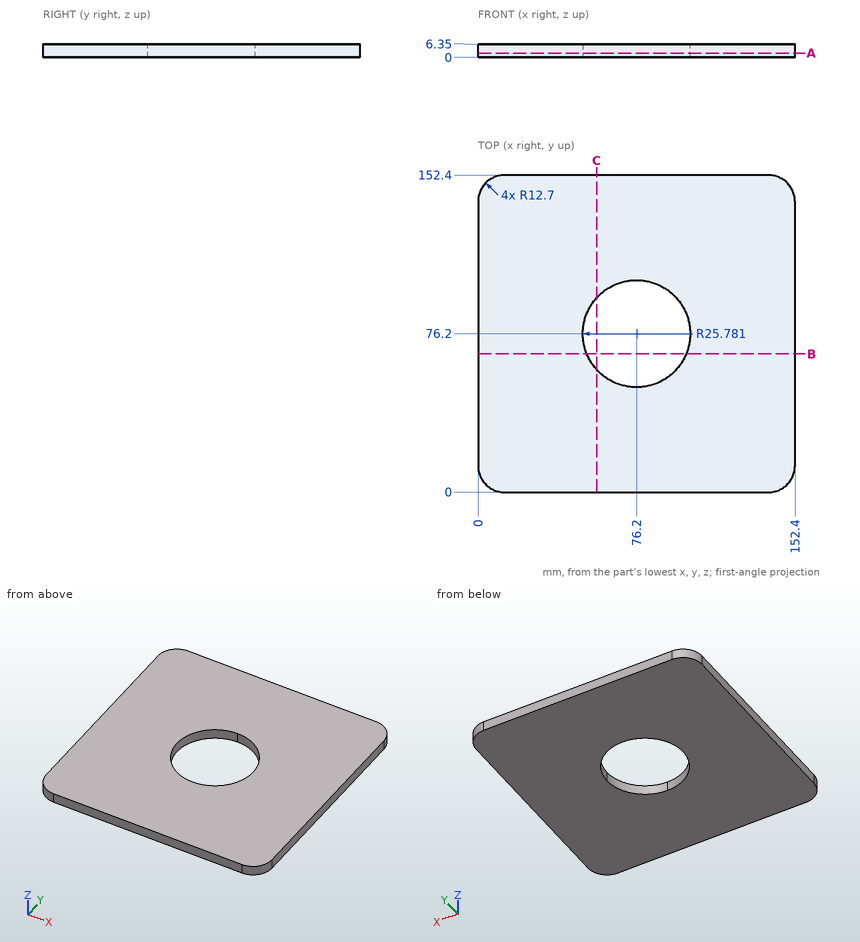
Answer from the drawing. Dimensions are ordinates in mm from the lowest x, y and z of the part. Coordinates: 2 decimals unless noted, no trailing zeros. Write each loop counter-clockwise with the first axis right and the second up, starting at its lowest first coordinate (ties: lowest second). Pieces come first, ordered by that corner, then holes. Notation, with made-up numbers: M 25,50.5 L 67,50.5 A7 cw 67,55.5 Z; hole C -21,5.5 d8. An arc over 180 degrees is marked long. Put each result on its own line as item: value. Start each with the question number.
1. A cutting plane is placed at A-A on z = 2. Write down the section's boundary in (x, y), then the cut area to 3 significant figures.
2. A cutting plane is placed at B-B on y = 66.5. Write down the section's boundary in (x, z), then the cut area to 3 significant figures.
3. Consider line 1 (X direction, y = 77, z = 1.75); line 2 (X direction, y = 92, z = 3.75); line 3 (Y direction, x = 58.5, z = 1.5). Determine where each line is inside the solid, lowest interval first. Write a range as from..to.
4. A flat-ended cylindrical pin translates along its axis: P1, Ø1, axis at x = 57, z = 0.5, coming from the -Y side. Find the tip coordinate at first contact, or state that the pin passes through.
5. A cutting plane is placed at C-C on x = 57. Write down the section's boundary in (y, z).
Resolved:
1. outline: M 0,12.7 A12.7 ccw 12.7,0 L 139.7,0 A12.7 ccw 152.4,12.7 L 152.4,139.7 A12.7 ccw 139.7,152.4 L 12.7,152.4 A12.7 ccw 0,139.7 Z; hole C 76.2,76.2 d51.56
1. area: 21,000 mm2
2. outline: M 0,0 L 52.31,0 L 52.31,6.35 L 0,6.35 Z; M 100.09,0 L 152.4,0 L 152.4,6.35 L 100.09,6.35 Z
2. area: 664 mm2
3. line 1: x = 0..50.43, 101.97..152.4
3. line 2: x = 0..55.83, 96.57..152.4
3. line 3: y = 0..57.46, 94.94..152.4
4. P1: stops at y = 0
5. outline: M 0,0 L 58.99,0 L 58.99,6.35 L 0,6.35 Z; M 93.41,0 L 152.4,0 L 152.4,6.35 L 93.41,6.35 Z
